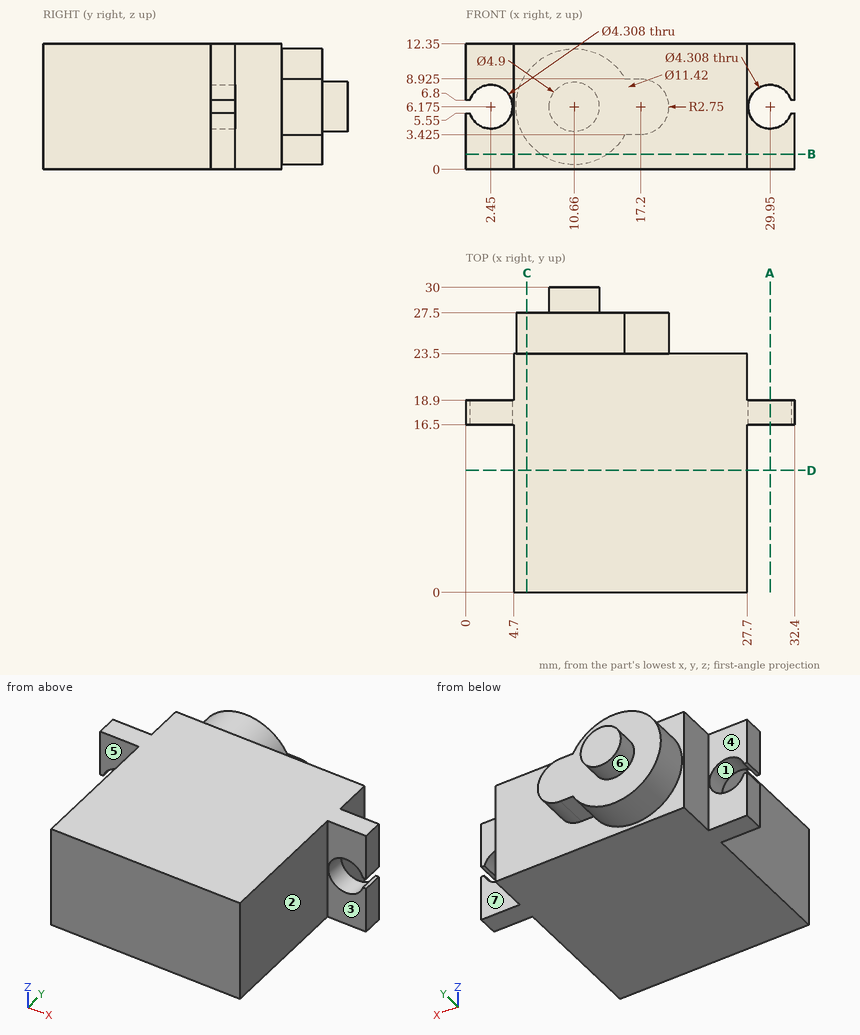
Verification items for this drawing (mm, ordinates from the low corner). A direction names the side the tool comes from. Give positions to 0.01 mm unless a question says otherwise; leave off trailing zeros. Loops run counter-clockwise (first coordinate to the right, second up) from the corner with the lowest first, then second, coordinate; pieces in that order, holes last.
(1) Release check for a two-part mould opening along X. For the marked faces 1, 2 and 3 record: released by +X, released by -X, zero draft, split by the parting line, or undercut.
From the geometry:
face 1: undercut
face 2: released by +X
face 3: zero draft
(2) Thickness scan on L1, parallel to Z at x = 29.95, y = 17.35; L2, parallel to Y at x = 16, z = 3.75; L3, parallel to Y at x = 23.5, z = 1.25. Record the ranges inside material, lowest first.
From the geometry:
L1: z = 0 to 4.02, 8.33 to 12.35
L2: y = 0 to 27.5
L3: y = 0 to 23.5
(3) Section check B-B on z = 1.5. Record the cut outline in (x, y), then the cut area to 3 significant figures.
From the geometry:
outline: (0, 16.5) - (4.7, 16.5) - (4.7, 0) - (27.7, 0) - (27.7, 16.5) - (32.4, 16.5) - (32.4, 18.9) - (27.7, 18.9) - (27.7, 23.5) - (13.94, 23.5) - (13.94, 27.5) - (7.38, 27.5) - (7.38, 23.5) - (4.7, 23.5) - (4.7, 18.9) - (0, 18.9) - close
area: 589 mm2
(4) Section check A-A on x = 29.95. Record the cut outline in (y, z).
From the geometry:
outline: (16.5, 0) - (18.9, 0) - (18.9, 4.02) - (16.5, 4.02) - close; (16.5, 8.33) - (18.9, 8.33) - (18.9, 12.35) - (16.5, 12.35) - close
(5) Section check C-C on x = 6. Record the cut outline in (y, z), then the cut area to 3 significant figures.
From the geometry:
outline: (0, 0) - (23.5, 0) - (23.5, 2.88) - (27.5, 2.88) - (27.5, 9.47) - (23.5, 9.47) - (23.5, 12.35) - (0, 12.35) - close
area: 317 mm2
(6) Section check D-D on y = 12. Record the cut outline in (x, z), then the cut area to 3 significant figures.
From the geometry:
outline: (4.7, 0) - (27.7, 0) - (27.7, 12.35) - (4.7, 12.35) - close
area: 284 mm2
(7) Set-up check for the marked faces 4, 5, 6 and 7: record each of +Z, -Z, +X, -X, +Y, -Y from which the full face is reachable in a straight line by a thin tool's end or side.
From the geometry:
face 4: +Z, -Z, -X, +Y
face 5: +Z, -Z, -X, -Y
face 6: +Y
face 7: +Z, -Z, +X, +Y
(8) Depth check by flat-ended pin: pin 1 Ø6 at (y, z) = (26, 8) entering from -X; pin 2 Ø2 at (x, z) = (19, 5) entering from +Y; pin 3 Ø1.4 at (x, z) = (1.5, 3.5) entering from -Y. Enter the tip coordinate at first touch or a pass-through.
From the geometry:
pin 1: stops at x = 4.7
pin 2: stops at y = 27.5
pin 3: stops at y = 16.5
